For this review, use the dimensioned drawing (mm, ordinates from the lowest corner) and the shaded views. A direction names the side the tool comes from. Give positions to 0.01 mm unless a question says otherwise; leave off trailing zeros. Loops run counter-clockwise (first coordinate to the right, second up) from the corner with the lowest first, then second, coordinate; pieces in that order, holes last. Notation, with made-up numbers: (38, -5.75) -> (84, -5.75) arc R15 ccw to (84, 8.25) -> close; hole circle Ø2 at (-8, 4). An arc over 180 degrees is marked (long way). Write each question's results on one line, items separated by ' | '. Start each with the question number.
Q1. Machinability: for the marked faces 1 and 2, which of the approach directions +Z, -Z, +X, -X, +Y, -Y give a long, thin tool a straight path to every point of the face, cutting with its end or side? Answer none if there is none.
Q2. Insertion check: pin 1 Ø4 at (x, y) = (19.5, 12.5) entering from +Z. The pin has a flat end and moves straight along its axis. Give the tip position at first contact, or say it passes through.
Q3. Mouldability with a two-part tool opening along Y and no side actions: class the marked faces 3, 4, 5 and 6 as released by +Y, released by -Y, zero draft, split by the parting line, or undercut.
Q4. We need section A-A (x = 20). Write out the cut boundary in (y, z) (1 decimal), plus the area to 3 significant figures.
Q5. We need section D-D (x = 10). Write out the cut boundary in (y, z), plus the area to 3 significant figures.
Q6. We need section C-C (y = 5.25). Write out the cut boundary in (x, z).
Q7. We need section B-B (y = 10). Write out the cut boundary in (x, z) (1 decimal), plus the area to 3 significant figures.
Q8. Wall thickness on L1, parallel to Y at x = 20, z = 63.5 (1 decimal); L2, parallel to Y at x = 23, z = 59.5 (1 decimal); L3, parallel to Z at x = 21, y = 9: over which ranges is each line inside the solid? List them lowest first. Write a range as [from, to].
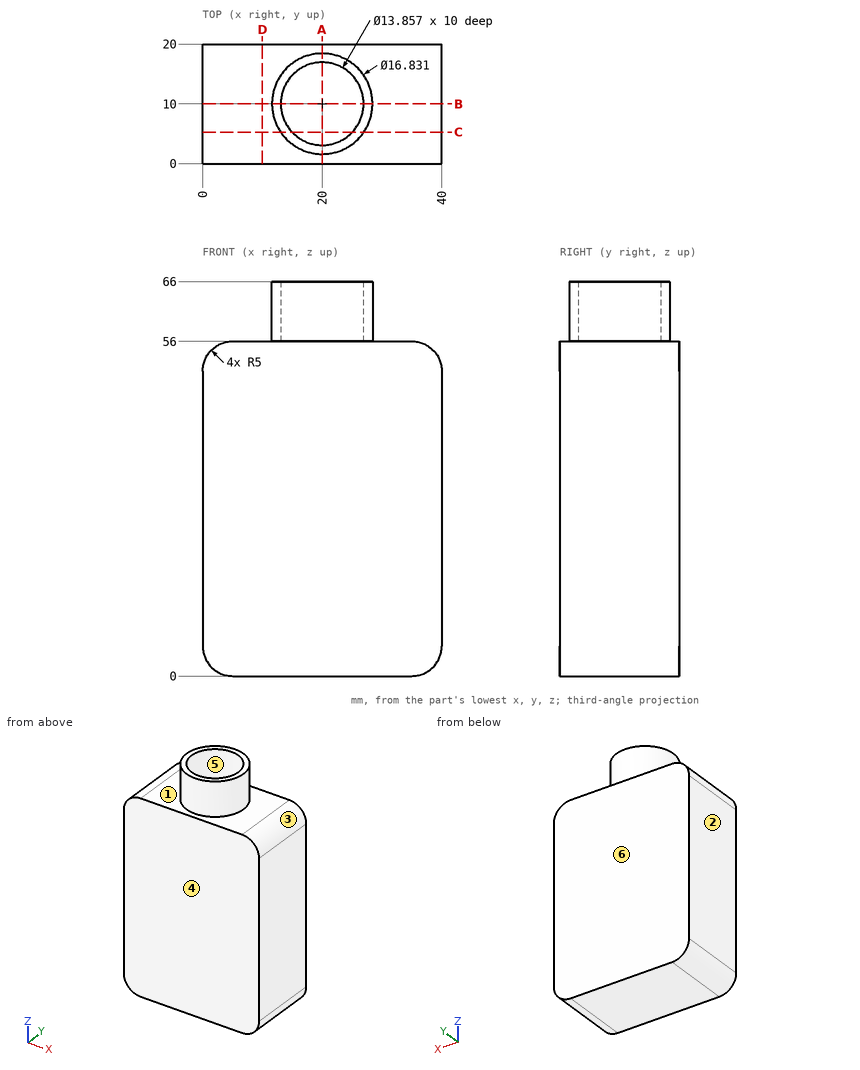
Output:
1) face 1: +Z | face 2: +Z, -Z, -X, +Y, -Y
2) pin 1: z = 56
3) face 3: zero draft | face 4: released by -Y | face 5: undercut | face 6: released by +Y
4) outline: (0, 0) -> (20, 0) -> (20, 56) -> (18.4, 56) -> (18.4, 66) -> (16.9, 66) -> (16.9, 56) -> (3.1, 56) -> (3.1, 66) -> (1.6, 66) -> (1.6, 56) -> (0, 56) -> close | area: 1,150 mm2
5) outline: (0, 0) -> (20, 0) -> (20, 56) -> (0, 56) -> close | area: 1,120 mm2
6) outline: (0, 5) arc R5 ccw to (5, 0) -> (35, 0) arc R5 ccw to (40, 5) -> (40, 51) arc R5 ccw to (35, 56) -> (26.95, 56) -> (26.95, 66) -> (25.04, 66) -> (25.04, 56) -> (14.96, 56) -> (14.96, 66) -> (13.05, 66) -> (13.05, 56) -> (5, 56) arc R5 ccw to (0, 51) -> close
7) outline: (0, 5) arc R5 ccw to (5, 0) -> (35, 0) arc R5 ccw to (40, 5) -> (40, 51) arc R5 ccw to (35, 56) -> (28.4, 56) -> (28.4, 66) -> (26.9, 66) -> (26.9, 56) -> (13.1, 56) -> (13.1, 66) -> (11.6, 66) -> (11.6, 56) -> (5, 56) arc R5 ccw to (0, 51) -> close | area: 2,250 mm2
8) L1: [1.6, 3.1], [16.9, 18.4] | L2: [2.1, 3.8], [16.2, 17.9] | L3: [0, 56]
